Verification items for the finished model (mm, model axes). A direction names the side the tool comes from. Coordinates: 2 decimals unless noted, no trailing zeros. Order: outer loops, then holes, each group sorted by start corner. A loop starts at its lowest first (then second) coordinate and runs counter-clockwise, first axis right, second up. Notation, with made-up numbers: M 64,19 L 70,19 A21 ccw 70,52 Z; hole C -39.75,21.5 d2. An arc over 180 degrees is marked long. Return JSON: item names as keys, results as strings. Group by question number.
1. Section check C-C, the plane x = -199.5. Record the cut outline in (y, z), plus the area to 3 significant figures.
2. Material ranges on line 1 along X through (y, z) = (269, 163); line 2 along Y through (x, z) = (-11, 116.5); line 3 along Z through (x, y) = (202, 258), recorded low to high.
3. Section check A-A, the plane z = 147. Record the cut outline in (x, y), plus the area to 3 significant figures.
4. Section check B-B, the plane y = 71. Record the cut outline in (x, z), plus the area to 3 significant figures.
5. Mould release check, pull along Y, two halves, no side actions. Record for faces 1 (the flat face through (-188, 304.8, 109)), 2 (the flat face through (-4, 323.85, 100)), 3 (the flat face through (-4, -323.85, 100)), 4 (the flat face through (196, 314, 25.4)): +Y half, -Y half, draft (parallel to the pull), parting line (faces both ways), or undercut.
6. Set-up check for faces 5 (the flat face through (-188, -4, 19.05)), 6 (the flat face through (-285.75, -5, 97)): record each of +Z, -Z, +X, -X, +Y, -Y from which the full face is reachable in a straight line by a thin tool's end or side.
7. Section check D-D, the plane x = 138. Record the cut outline in (y, z).
8. Gauge pin test, flat end, axial feed: pin 1 (1.5 mm diameter, centred on x = -72, y = -41, fed in from +Z). Record the tip position at first contact, or that the pin passes through.
```python
from build123d import *

# Parameters (mm, degrees)
F0_W          = 571.5
F0_H          = 196.85
F1_DEPTH      = 323.85
F2_T          = -19.05
F4_DEPTH      = 647.701
F5_W          = 19.05
F5_H          = 177.8
F6_DEPTH      = 304.8
F6_DEPTH_BACK = 304.8


with BuildPart() as f1:
    # F0 (on Front) → F1 (new body, symmetric)
    with BuildSketch(Plane.XZ):
        with Locations((0, 98.425)):
            Rectangle(F0_W, F0_H)
    extrude(amount=F1_DEPTH, both=True)

    # F2
    f2_openings = [f1.faces().sort_by_distance(p)[0] for p in [
        (0, 0, 196.85),
    ]]
    offset(amount=F2_T, openings=f2_openings)

    # F3 (on face) → F4 (cut, through all)
    with BuildSketch(Plane.XZ.offset(323.85)):
        with BuildLine():
            Line((-234.4171066227, 25.4), (-159.2828933773, 25.4))
            ThreePointArc((-159.2828933773, 25.4), (-196.85, 57.15), (-234.4171066227, 25.4))
        make_face()
        with BuildLine():
            Line((-37.5671066227, 25.4), (37.5671066227, 25.4))
            ThreePointArc((37.5671066227, 25.4), (0, 57.15), (-37.5671066227, 25.4))
        make_face()
        with BuildLine():
            ThreePointArc((234.4171066227, 25.4), (196.85, 57.15), (159.2828933773, 25.4))
            Line((159.2828933773, 25.4), (234.4171066227, 25.4))
        make_face()
    extrude(amount=-F4_DEPTH, mode=Mode.SUBTRACT)

    # F5 (on Front) → F6 (join, two sides)
    with BuildSketch(Plane.XZ) as f6_sk:
        with Locations((-98.425, 107.95)):
            Rectangle(F5_W, F5_H)
        with Locations((98.425, 107.95)):
            Rectangle(F5_W, F5_H)
    extrude(amount=F6_DEPTH)
    extrude(f6_sk.sketch, amount=-F6_DEPTH_BACK)


solid = f1.part
```
Answers follow:
{
 "1": {"outline": "M -323.85,0 L 323.85,0 L 323.85,25.4 L 304.8,25.4 L 304.8,19.05 L -304.8,19.05 L -304.8,25.4 L -323.85,25.4 Z; M -323.85,57.06 L -304.8,57.06 L -304.8,196.85 L -323.85,196.85 Z; M 304.8,57.06 L 323.85,57.06 L 323.85,196.85 L 304.8,196.85 Z", "area": "17,900 mm^2"},
 "2": {"line 1": "-285.75 to -266.7, -107.95 to -88.9, 88.9 to 107.95, 266.7 to 285.75", "line 2": "-323.85 to -304.8, 304.8 to 323.85", "line 3": "0 to 19.05"},
 "3": {"outline": "M -285.75,-323.85 L 285.75,-323.85 L 285.75,323.85 L -285.75,323.85 Z; hole M -266.7,-304.8 L -107.95,-304.8 L -107.95,304.8 L -266.7,304.8 Z; hole M -88.9,-304.8 L 88.9,-304.8 L 88.9,304.8 L -88.9,304.8 Z; hole M 107.95,-304.8 L 266.7,-304.8 L 266.7,304.8 L 107.95,304.8 Z", "area": "68,200 mm^2"},
 "4": {"outline": "M -285.75,0 L 285.75,0 L 285.75,196.85 L 266.7,196.85 L 266.7,19.05 L 107.95,19.05 L 107.95,196.85 L 88.9,196.85 L 88.9,19.05 L -88.9,19.05 L -88.9,196.85 L -107.95,196.85 L -107.95,19.05 L -266.7,19.05 L -266.7,196.85 L -285.75,196.85 Z", "area": "24,400 mm^2"},
 "5": {"face 1": "undercut", "face 2": "+Y half", "face 3": "-Y half", "face 4": "draft"},
 "6": {"face 5": "+Z", "face 6": "+Z, -Z, -X, +Y, -Y"},
 "7": {"outline": "M -323.85,0 L 323.85,0 L 323.85,196.85 L 304.8,196.85 L 304.8,19.05 L -304.8,19.05 L -304.8,196.85 L -323.85,196.85 Z"},
 "8": {"pin 1": "z = 19.05"}
}
